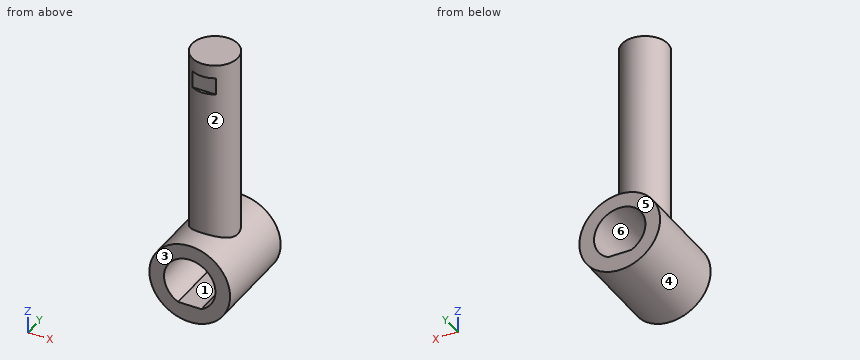
from build123d import *

# Parameters (mm, degrees)
SKETCH2_R               = 6.25
BOSS_EXTRUDE3_DEPTH     = 60
SKETCH1_R               = 11
BOSS_EXTRUDE4_DEPTH     = 12.5
CUT_EXTRUDE1_DEPTH      = 63.267567936
CUT_EXTRUDE1_DEPTH_BACK = 63.267567936
CUT_EXTRUDE2_DEPTH      = 2.35


with BuildPart() as part:
    # Sketch2 → Boss-Extrude3 (new body)
    with BuildSketch(Plane.XY):
        Circle(SKETCH2_R)
    extrude(amount=BOSS_EXTRUDE3_DEPTH)

    # Sketch1 → Boss-Extrude4 (add, symmetric)
    with BuildSketch(Plane(origin=(0, 0, 0), x_dir=(1, 0, 0), z_dir=(0, 1, 0))):
        with Locations(Location((0, 0, 0), (0, 0, 270))):
            Circle(SKETCH1_R)
    extrude(amount=BOSS_EXTRUDE4_DEPTH, both=True)

    # Sketch1_4 → Cut-Extrude1 (cut, two sides: drawn at the far end of the back side and taken through both)
    with BuildSketch(Plane(origin=(0, 0, 0), x_dir=(1, 0, 0), z_dir=(0, 1, 0)).offset(-CUT_EXTRUDE1_DEPTH_BACK)):
        with BuildLine():
            Line((3.175, 6.238539493), (-3.175, 6.238539493))
            ThreePointArc((-3.175, 6.238539493), (0, -7), (3.175, 6.238539493))
        make_face()
    extrude(amount=CUT_EXTRUDE1_DEPTH + CUT_EXTRUDE1_DEPTH_BACK, mode=Mode.SUBTRACT)

    # Sketch3 → Cut-Extrude2 (cut, symmetric)
    with BuildSketch(Plane.XY.offset(54)):
        with BuildLine():
            Line((-3.175, -5.38348168), (3.175, -5.38348168))
            ThreePointArc((3.175, -5.38348168), (0, -6.25), (-3.175, -5.38348168))
        make_face()
    extrude(amount=CUT_EXTRUDE2_DEPTH, both=True, mode=Mode.SUBTRACT)


solid = part.part
Could you check a few things on this model? Use its own coordinates, in mm. Face numbers are marked on the shaded views. A direction names the side the tool comes from. Coordinates: 2 decimals unless noted, no trailing zeros. Order: outer loops, then holes, each group sorted by start corner. A loop starts at its lowest first (then second) coordinate and runs counter-clockwise, first axis right, second up. Notation, with made-up numbers: (84.25, 51.5) - (91.25, 51.5) arc R29 ccw to (91.25, 88.5) - close; hole circle Ø3 at (32.5, 76). An arc over 180 degrees is marked (long way). Answer in a Markdown table with one row per item. Add a question column.
(1) Will these pins go through, and if not, where does the flat tip stop? pin 1 (12 mm diameter, centred on x = 2.5, z = 26, fed in from +Y); pin 2 (10 mm diameter, centred on x = -2.5, z = 39, fed in from -Y); pin 3 (3 mm diameter, centred on x = -6.5, z = 46, fed in from -Y).
(2) I need wall thicknesses on L1, parallel to X at y = -7.5, z = 0; L2, parallel to X at y = -5.75, z = -6; L3, parallel to Z at x = 2.5, y = 1. Which ranges of each line are inside material? Lowest first, please.
(3) If we section it at A-A, the plane x = 0: Please give me the cut outline in (y, z), then the cut area to 3 significant figures.
(4) If we mould it in two halves opening along X, with no side actions, what happens to the marked faces 4, 5 and 6? For each: released by +X, released by -X, zero draft, split by the parting line, or undercut.
(5) If we section it at B-B, the plane z = 0: Please give me the cut outline in (x, y).
(6) If we section it at C-C, the plane y = 0: Please give me the cut outline in (x, z) (3 decimals), then the cut area to 3 significant figures.
(7) On a 3-axis mill with a long thin cutter (end or side, diameter ignored), from which of +Z, -Z, +X, -X, +Y, -Y can I reach the whole of each face in a straight line? I mean the marked faces 1, 2 and 3. Say none if no direction works.
(8) If we section it at D-D, the plane x = -5.25: Please give me the cut outline in (y, z), then the cut area to 3 significant figures.
Results are:
| question | item | result |
|---|---|---|
| 1 | pin 1 | stops at y = 6.25 |
| 1 | pin 2 | stops at y = -6.25 |
| 1 | pin 3 | stops at y = -3.75 |
| 2 | L1 | x = -11 to -7, 7 to 11 |
| 2 | L2 | x = -9.22 to -3.61, 3.61 to 9.22 |
| 2 | L3 | z = -10.71 to -6.24, 6.54 to 60 |
| 3 | outline | (-12.5, -11) - (12.5, -11) - (12.5, -6.24) - (-12.5, -6.24) - close; (-12.5, 7) - (12.5, 7) - (12.5, 11) - (6.25, 11) - (6.25, 60) - (-6.25, 60) - (-6.25, 56.35) - (-5.38, 56.35) - (-5.38, 51.65) - (-6.25, 51.65) - (-6.25, 11) - (-12.5, 11) - close |
| 3 | area | 827 mm2 |
| 4 | face 4 | split by the parting line |
| 4 | face 5 | zero draft |
| 4 | face 6 | undercut |
| 5 | outline | (-11, -12.5) - (-7, -12.5) - (-7, 12.5) - (-11, 12.5) - close; (7, -12.5) - (11, -12.5) - (11, 12.5) - (7, 12.5) - close |
| 6 | outline | (-6.25, 9.052) arc R11 ccw (long way) to (6.25, 9.052) - (6.25, 60) - (-6.25, 60) - close; hole (-3.175, -6.239) - (3.175, -6.239) arc R7 ccw (long way) to start |
| 6 | area | 850 mm2 |
| 7 | face 1 | +Y, -Y |
| 7 | face 2 | +Z |
| 7 | face 3 | +Z, -Z, +X, -X, -Y |
| 8 | outline | (-12.5, -9.67) - (12.5, -9.67) - (12.5, -4.63) - (-12.5, -4.63) - close; (-12.5, 4.63) - (12.5, 4.63) - (12.5, 9.67) - (3.39, 9.67) - (3.39, 60) - (-3.39, 60) - (-3.39, 9.67) - (-12.5, 9.67) - close |
| 8 | area | 593 mm2 |
